Geometry: see drawing. Coordinates: mm, zero at the bounding-box minimum. A direction names the side the tool comes from. Give positions to 0.01 mm unless a question says otherwise; leave off trailing zeros. Loops run counter-clockwise (first coordinate to the right, second up) from the corner with the lowest first, then second, coordinate; pieces in that order, holes last. Notation, with made-up numbers: (60.5, -4) - (112.5, -4) arc R11 cw to (112.5, 3) - close; hole circle Ø4 at (13, 25). An arc over 180 degrees is marked (long way). Use one line per item in the form item = value.
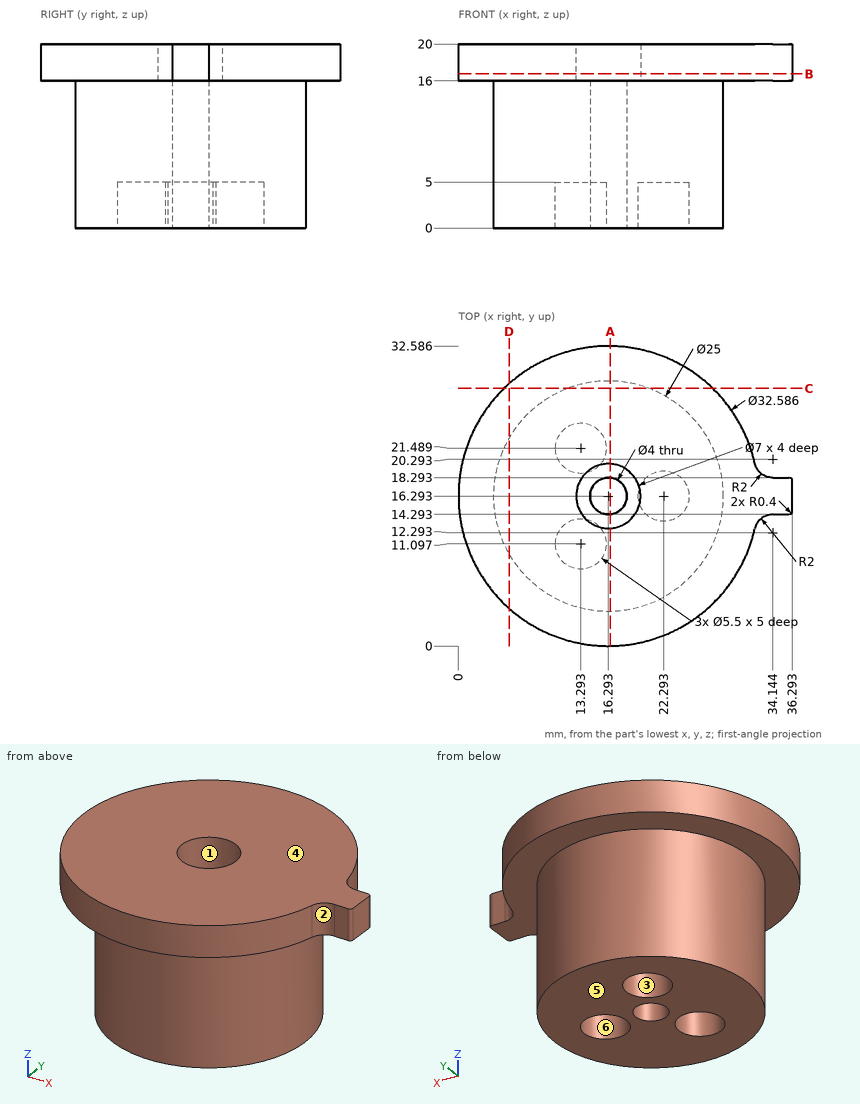
(1) Cut plane D-D (x = 5.5). Return the cut outline in (y, z), plus the area to 3 significant figures.
Solution:
outline = (4.09, 16) - (9.99, 16) - (9.99, 0) - (22.6, 0) - (22.6, 16) - (28.5, 16) - (28.5, 20) - (4.09, 20) - close
area = 299 mm2
(2) Pin query (flat end, axial travel): P1, Ø3, axis at x = 10.5, z = 9, coming from the +Y side; P2, Ø0.5, axis at x = 35.5, z = 17.5, coming from the +Y side; P3, Ø5, axis at x = 16.29, y = 16.29, coming from the +Z side; P4, Ø4, axis at x = 31, z = 3, coming from the +Y side. Return the tip coordinate at first contact, or that it passes through.
Solution:
P1 = 28.03
P2 = 18.29
P3 = 16
P4 = through
(3) Material intervals for L1, parallel to X at y = 15, z = 14 (1 decimal); L2, parallel to Z at x = 30, y = 19.5; L3, parallel to X at y = 25, z = 7.75 (1 decimal), sorted ascending. Write a range as from..to.
Solution:
L1 = 3.9..14.8, 17.8..28.7
L2 = 16..20
L3 = 7.3..25.3
(4) Cut plane B-B (z = 16.75). Return the cut outline in (x, y).
Solution:
outline = (32.19, 12.73) arc R2 cw to (34.14, 14.29) - (35.89, 14.29) arc R0.4 ccw to (36.29, 14.69) - (36.29, 17.89) arc R0.4 ccw to (35.89, 18.29) - (34.14, 18.29) arc R2 cw to (32.19, 19.86) arc R16.29 ccw (long way) to start; hole circle Ø7 at (16.29, 16.29)
(5) Access query for the marked faces 5 and 6. Directions: +Z, -Z, +X, -X, +Y, -Y. A direction counts if a zero-diameter tool reaches every point of the face in a straight line with its end or side. Return the directions, or none.
Solution:
face_5 = -Z, +X, -X, +Y, -Y
face_6 = -Z
(6) Pull-direction query (Y, two-part tool) for the marked faces 1, 2, 3 and 4; classes: released by +Y, released by -Y, zero draft, split by the parting line, or undercut.
Solution:
face_1 = undercut
face_2 = released by -Y
face_3 = undercut
face_4 = zero draft
(7) Cut plane C-C (y = 28). Return the cut outline in (x, z) (1 decimal).
Solution:
outline = (5, 16) - (11.9, 16) - (11.9, 0) - (20.7, 0) - (20.7, 16) - (27.6, 16) - (27.6, 20) - (5, 20) - close
(8) Cut plane A-A (x = 16.5). Return the cut outline in (y, z) (1 decimal).
Solution:
outline = (0, 16) - (3.8, 16) - (3.8, 0) - (14.3, 0) - (14.3, 16) - (12.8, 16) - (12.8, 20) - (0, 20) - close; (18.3, 0) - (28.8, 0) - (28.8, 16) - (32.6, 16) - (32.6, 20) - (19.8, 20) - (19.8, 16) - (18.3, 16) - close
